```python
from build123d import *

# Parameters (mm, degrees)
F1_DEPTH = 20
F2_R     = 3
F3_R     = 1.5
F4_DEPTH = 25


with BuildPart() as f1:
    # F0 (on Top) → F1 (new body)
    with BuildSketch(Plane.XY):
        Polygon((0, 5.021903), (0, 0), (0, -3.424607), (15.019838, -3.424607), (15.019838, 5.021903), align=None)
        Polygon((0, -3.424607), (0, 0), (0, 5.021903), (0, 13.150787), (0, 20), (14.283885, 20), (27.16307, 20), (27.16307, 30), (14.283885, 30), (-10.716115, 30), (-10.716115, 29), (-10.716115, -21), (-10.716115, -29.918844), (0, -29.918844), (0, -21), (0, -20), (0, -8.509332), align=None)
    extrude(amount=F1_DEPTH)

    # F2
    f2_edges = [f1.edges().sort_by_distance(p)[0] for p in [
        (13.581535, 20, 0),
        (27.16307, 25, 0),
        (8.223477, 30, 0),
        (-10.716115, 0.040578, 0),
        (-5.358057, -29.918844, 0),
        (0, -16.671725, 0),
        (7.509919, -3.424607, 0),
        (15.019838, 0.798648, 0),
        (7.509919, 5.021903, 0),
        (0, 12.510952, 0),
        (27.16307, 20, 10),
        (27.16307, 30, 10),
        (27.16307, 25, 20),
        (15.019838, -3.424607, 10),
        (15.019838, 5.021903, 10),
        (15.019838, 0.798648, 20),
        (-5.358057, -29.918844, 20),
        (-10.716115, -29.918844, 10),
        (0, -29.918844, 10),
        (13.581535, 20, 20),
        (0, 12.510952, 20),
        (8.223477, 30, 20),
        (-10.716115, 0.040578, 20),
        (0, -16.671725, 20),
        (7.509919, -3.424607, 20),
        (7.509919, 5.021903, 20),
    ]]
    fillet(f2_edges, radius=F2_R)

    # F3 (on face) → F4 (cut)
    with BuildSketch(Plane.XY.offset(20)):
        with Locations((-5.009224, 24.547122)):
            Circle(F3_R)
    extrude(amount=-F4_DEPTH, mode=Mode.SUBTRACT)


solid = f1.part
```
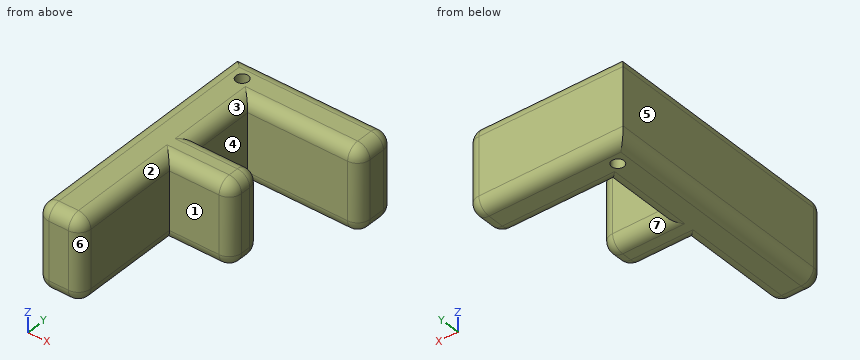
Geometry check sheet. Reference: the model listing, model coordinates, mm. Face numbers are marked on the shaded views. A direction names the side the tool comes from. Coordinates: 2 decimals unless noted, no trailing zeros. Order: outer loops, then holes, each group sorted by start corner. A loop starts at its lowest first (then second) coordinate and runs counter-clockwise, first axis right, second up. Notation, with made-up numbers: M 23.25,25.5 L 36.25,25.5 A17 ccw 36.25,41.5 Z; hole C 1.5,35 d1. An arc over 180 degrees is marked long. One line per question, with ' | ' between items. Start each with the question number.
Item 1: Cross-section at D-D on x = 23. Enter the section's corners in (y, z), then the cut area to 3 significant figures.
Item 2: Material ranges on L1, parallel to Y at x = 8, z = 17.25; L2, parallel to Y at x = 14, z = 14.5; L3, parallel to X at y = 12.5, z = 17.25, recorded low to high. Write a range as [from, to].
Item 3: Cross-section at B-B on y = 8. Enter the section's corners in (x, z).
Item 4: Gauge pin test, flat ends, axial feed: pin 1 (2 mm diameter, centred on y = 4, z = 16.5, fed in from +X); pin 2 (3 mm diameter, centred on x = 6.5, z = 13.5, fed in from -Y); pin 3 (4 mm diameter, centred on x = -2.5, z = 17, fed in from -Y); pin 4 (11 mm diameter, centred on y = -17, z = 8.5, fed in from +X). Record the tip position at first contact, or that the pin passes through.
Item 5: Draft check along Y on the marked faces 5, 6 and 7. Enter one of: pulls with the +Y half, pulls with the -Y half, needs draft (parallel to the pull), parting line crosses it, or undercut.
Item 6: Cross-section at A-A on x = 4.5. Enter the section's corners in (y, z).
Item 7: Set-up check for the marked faces 1, 2, 3 and 4: record each of +Z, -Z, +X, -X, +Y, -Y from which the full face is reachable in a straight line by a thin tool's end or side.
Item 8: Cross-section at C-C on z = 7.25. Enter the section's corners in (x, y).
Findings:
1) outline: M 20,3 A3 ccw 23,0 L 27,0 A3 ccw 30,3 L 30,17 A3 ccw 27,20 L 23,20 A3 ccw 20,17 Z | area: 192 mm²
2) L1: y = [-3.41, 5.01], [20.01, 29.99] | L2: y = [-2.68, 4.28], [20, 30] | L3: x = [-10.71, -0.01]
3) outline: M -10.72,3 A3 ccw -7.72,0 L -3,0 A3 ccw 0,3 L 0,17 A3 ccw -3,20 L -7.72,20 A3 ccw -10.72,17 Z
4) pin 1: stops at x = 14.86 | pin 2: stops at y = -3.42 | pin 3: stops at y = -29.92 | pin 4: stops at x = 0
5) face 5: needs draft | face 6: pulls with the -Y half | face 7: undercut
6) outline: M -3.42,3 A3 ccw -0.42,0 L 2.02,0 A3 ccw 5.02,3 L 5.02,17 A3 ccw 2.02,20 L -0.42,20 A3 ccw -3.42,17 Z; M 20,3 A3 ccw 23,0 L 27,0 A3 ccw 30,3 L 30,17 A3 ccw 27,20 L 23,20 A3 ccw 20,17 Z
7) face 1: +Z, -Z, +X, -Y | face 2: +Z, +X, -Y | face 3: +Z, +X | face 4: +Z, -Z, +X
8) outline: M -10.72,-26.92 A3 ccw -7.72,-29.92 L -3,-29.92 A3 ccw 0,-26.92 L 0,-3.42 L 12.02,-3.42 A3 ccw 15.02,-0.42 L 15.02,2.02 A3 ccw 12.02,5.02 L 0,5.02 L 0,20 L 24.16,20 A3 ccw 27.16,23 L 27.16,27 A3 ccw 24.16,30 L -10.72,30 Z; hole C -5.01,24.55 d3
